```python
from build123d import *

# Parameters (mm, degrees)
SKETCH1_R   = 25
SKETCH1_R_2 = 19.9
BODY_DEPTH  = 406
SKETCH2_W   = 2
SKETCH2_H   = 2.1


with BuildPart() as part:
    # Sketch1 → Body (new body)
    with BuildSketch(Plane.XY):
        with Locations(Location((0, 0, 0), (0, 0, 180))):
            Circle(SKETCH1_R)
        with Locations(Location((0, 0, 0), (0, 0, 180))):
            Circle(SKETCH1_R_2, mode=Mode.SUBTRACT)
    extrude(amount=BODY_DEPTH)

    # Sketch2 → Ret Ring Grooves (revolve, cut)
    with BuildSketch(Plane(origin=(0, 0, 0), x_dir=(0, 0, -1), z_dir=(1, 0, 0)), mode=Mode.PRIVATE) as ret_ring_grooves_sk:
        with Locations((-403, 23.95)):
            Rectangle(SKETCH2_W, SKETCH2_H)
        with Locations((-361, 23.95)):
            Rectangle(SKETCH2_W, SKETCH2_H)
        with Locations((-55.5, 23.95)):
            Rectangle(SKETCH2_W, SKETCH2_H)
        with Locations((-350.5, 23.95)):
            Rectangle(SKETCH2_W, SKETCH2_H)
        with Locations((-45, 23.95)):
            Rectangle(SKETCH2_W, SKETCH2_H)
        with Locations((-3, 23.95)):
            Rectangle(SKETCH2_W, SKETCH2_H)
    revolve(ret_ring_grooves_sk.sketch.rotate(Axis((0, 0, 0), (0, 0, 1)), 90), axis=Axis((0, 0, 0), (0, 0, 1)), mode=Mode.SUBTRACT)


solid = part.part
```
Geometry check sheet. Reference: the model listing, model coordinates, mm. A direction names the side the tool comes from. Coordinates: 2 decimals unless noted, no trailing zeros. Order: outer loops, then holes, each group sorted by start corner. A loop starts at its lowest first (then second) coordinate and runs counter-clockwise, first axis right, second up.
Q1. Draft check along X on faces 1 (the face through (17, 11, 0)), 2 (the face through (4.964, 22.355, 2.986)), 3 (the face through (15.8, 12.1, 200.2)). Enter one of: released by +X, released by -X, zero draft, split by the parting line, or undercut.
Reply:
face 1: zero draft
face 2: split by the parting line
face 3: undercut
Q2. Tool access check on faces 4 (the face through (11, 20.3, 2)), 5 (the face through (-23.846, -7.509, 200.949)). Record the directions out of +Z, -Z, +X, -X, +Y, -Y that give a thin tool (end or side, any length) a straight path to the whole face; none if there is none.
Reply:
face 4: none
face 5: +Z, -Z
Q3. Depth check by flat-ended pin: pin 1 Ø5 at (x, z) = (9.5, 84.5) entering from +Y; pin 2 Ø12 at (y, z) = (-11, 53) entering from -X; pin 3 Ø5 at (x, z) = (19, 81.5) entering from -Y. Enter the tip coordinate at first touch or a pass-through.
Reply:
pin 1: stops at y = 24
pin 2: stops at x = -24.49
pin 3: stops at y = -18.78
Q4. Thickness scan on probe 1 along Y at (x, z) = (1.5, 286.5); probe 2 along Y at (x, z) = (0, 92); probe 3 along X at (y, z) = (1, 97). Record the ranges inside material, lowest first.
Reply:
probe 1: y = -24.95 to -19.84, 19.84 to 24.95
probe 2: y = -25 to -19.9, 19.9 to 25
probe 3: x = -24.98 to -19.87, 19.87 to 24.98
Q5. Sectioned sample at A-A on z = 95. Record the cut outline in (x, y), and give its area (3 significant figures).
Reply:
outline: circle Ø50 at (0, 0); hole circle Ø39.8 at (0, 0)
area: 719 mm2
